Work out the finished part from the listing and answer in its coordinate system (mm). A direction names the side the tool comes from. Give positions to 0.01 mm unless a question says otherwise; leave off trailing zeros. Loops run counter-clockwise (first coordinate to the right, second up) from the corner with the lowest first, then second, coordinate; pieces in that order, holes last. Notation, with made-up numbers: (10, 68.5) - (39, 68.5) arc R9 ccw to (39, 78.5) - close; hole circle Ø4 at (63, 24). An arc over 180 degrees is marked (long way). One line per question, with ' | ' between items. Start each with the question number.
1. Which of the six approach directions +Z, -Z, +X, -X, +Y, -Y give full straight-line access (tool end or side, diameter ignored) to faces 4 (the face through (-195, 202.448, -136)), 5 (the face through (-218.044, 200.355, -68.665)), 6 (the face through (228.932, 150.636, 103.963))?
2. Section A-A (z = 0) is taken. Determine the outline of the cut face in (x, y).
3. Section D-D (z = 82.5) is taken. Determine the outline of the cut face in (x, y).
4. Section C-C (y = 323.5) is taken. Determine the outline of the cut face in (x, z).
5. Each of these flat-tipped pins is pushed along its axis until it touches: pin 1 (3 mm diameter, centred on x = 98.5, z = 5.5, fed in from +Y); pin 2 (22.5 mm diameter, centred on y = 235, z = -180, fed in from -X) (3 decimals); pin 3 (2 mm diameter, centred on x = -194.5, y = 75.5, fed in from +Z). Where does it stop, or does it pass through?
6. Find the intervals of material crossed by line 1 (X direction, y = 276, z = 0); line 2 (Y direction, x = -199, z = -149), in increasing order.
7. Section B-B (x = 0) is taken. Determine the outline of the cut face in (y, z), plus the area to 3 significant figures.
8. For a pull along Z with two mould halves and no side action, classify faces 1 (the face through (-223.75, 226.65, -76.73)), 2 (the face through (-161.211, 227.742, -195.512)), 3 (the face through (-4, -25.4, 4)) as released by +Z, released by -Z, zero draft, split by the parting line, or undercut.
Autodesk Inventor part; units mm, degrees
ref_plane "Work Plane1" through (-254, 0, 0) normal (1, 0, 0) x (0, 1, 0)
ref_plane "XZ Plane" through (0, 0, 0) normal (0, 1, 0) x (-1, 0, 0)
ref_plane "XY Plane" through (0, 0, 0) normal (0, 0, 1) x (1, 0, 0)
sketch "Sketch1" plane through (0, 0, 0) normal (0, 1, 0) x (-1, 0, 0)
  circle A0 centre (0, 0) radius 228.6
  circle A1 centre (0, 0) radius 254
  dimension "d0" = 457.2
  dimension "d1" = 508
extrude "Extrusion1" add sketch "Sketch1" along normal blind 406.4
sketch "Sketch2" plane through (0, 0, 0) normal (0, -1, 0) x (1, 0, 0)
  circle A0 centre (0, 0) radius 254
extrude "Extrusion2" add sketch "Sketch2" along normal blind 25.4
ref_plane "Work Plane1" through (-254, 0, 0) normal (1, 0, 0) x (0, 1, 0)
sketch "Sketch3" plane through (-254, 0, 0) normal (1, 0, 0) x (0, 1, 0)
  line L0 (227.1973, -170.7692) -> (227.1973, -101.4716) construction
  line L1 (251.9465, -170.7692) -> (251.9465, -101.4716)
  line L2 (202.4481, -101.4716) -> (202.4481, -170.7692)
  arc A0 (202.4481, -170.7692) -> (251.9465, -170.7692) centre (227.1973, -170.7692) ccw
  arc A1 (251.9465, -101.4716) -> (202.4481, -101.4716) centre (227.1973, -101.4716) ccw
  point P0 (0, 0)
  point P1 (227.1973, -136.1204)
extrude "Extrusion3" cut sketch "Sketch3" along normal blind 98.425
ref_plane "Plane for hole making" through (254, 0, 0) normal (1, 0, 0) x (0, 1, 0)
sketch "Sketch4" plane through (254, 0, 0) normal (1, 0, 0) x (0, 1, 0)
  point P0 (0, 0)
sketch "Sketch5" plane through (254, 0, 0) normal (1, 0, 0) x (0, 1, 0)
  circle A0 centre (164.2862, 0) radius 104.8554
  point P0 (0, 0)
extrude "Extrusion4" cut sketch "Sketch5" against normal blind 76.2
Conclusion:
1) face 4: -X | face 5: +Y | face 6: +X
2) outline: (-254, -25.4) - (254, -25.4) - (254, 59.43) - (228.6, 59.43) - (228.6, 0) - (-228.6, 0) - (-228.6, 406.4) - (-254, 406.4) - close; (228.6, 269.14) - (254, 269.14) - (254, 406.4) - (228.6, 406.4) - close
3) outline: (-240.23, -25.4) - (240.23, -25.4) - (240.23, 99.57) - (213.19, 99.57) - (213.19, 0) - (-213.19, 0) - (-213.19, 406.4) - (-240.23, 406.4) - close; (213.19, 229) - (240.23, 229) - (240.23, 406.4) - (213.19, 406.4) - close
4) outline: circle Ø508 at (0, 0); hole circle Ø457.2 at (0, 0)
5) pin 1: y = 0 | pin 2: x = -155.575 | pin 3: z = 164.54
6) line 1: -254 to -228.6, 228.6 to 254 | line 2: -25.4 to 202.45, 251.95 to 406.4
7) outline: (-25.4, -254) - (406.4, -254) - (406.4, -228.6) - (0, -228.6) - (0, 228.6) - (406.4, 228.6) - (406.4, 254) - (-25.4, 254) - close | area: 33,500 mm²
8) face 1: released by -Z | face 2: undercut | face 3: zero draft
